Geometry check sheet. Reference: the model listing, model coordinates, mm. Face numbers are marked on the shaded views. A direction names the side the tool comes from. Give positions to 0.01 mm unless a question says otherwise; leave off trailing zeros. Order: outer loops, then holes, each group sorted by start corner. A loop starts at its lowest first (then second) coordinate and runs counter-clockwise, first axis right, second up. Notation, with made-up numbers: M 76.25,-9 L 87.25,-9 A17 ccw 87.25,9 Z; hole C 5,52.5 d10. An arc over 180 degrees is marked long. Put each result on its own line as item: value. Start each with the question number.
Q1. Material ranges on L1, parallel to Y at x = 0, z = 4.75; L2, parallel to Y at x = -2, z = 4.5; L3, parallel to X at y = 1, z = 4.25, recorded low to high.
Q2. Mould release check, pull along X, two halves, no side actions. Record for the marked faces 3, 4 and 5: +X half, -X half, draft (parallel to the pull), parting line (faces both ways), or undercut.
Q3. Section check B-B on y = 0. Record the cut outline in (x, z).
Q4. Access from +Z, -Z, +X, -X, +Y, -Y to the whole of each face (thin tool, end or side, straight path). Record for the marked faces 1 and 2.
Q5. Go/stop test with flat-tipped pins: pin 1 (5 mm diameter, centred on x = -5, z = 2.5, fed in from -Y); pin 2 (1.5 mm diameter, centred on y = 1, z = 3, fed in from -X); pin 3 (4 mm diameter, centred on x = 4, y = 4.5, fed in from +Z). Record where each tip stops, or that it passes through.
Q6. Section check D-D on z = 20. Record the cut outline in (x, y).
Q7. Section check A-A on z = 7.75. Record the cut outline in (x, y).
```python
from build123d import *

# Parameters (mm, degrees)
F0_R     = 5.25
F1_DEPTH = 11.7
F2_R     = 8.9
F3_DEPTH = 1.5
F4_R     = 3.4
F5_DEPTH = 9.5
F7_R     = 0.0965685425
F8_R     = 3.4
F9_DEPTH = 11.8
F10_R    = 1.4485281374


# Not quite as in the source:
# - a fillet or chamfer that OpenCascade refuses, or shapes differently, is made with other operations: its cross-section is extruded or revolved along the edge and cut away or added


with BuildPart() as f1:
    # F0 (on Top) → F1 (new body)
    with BuildSketch(Plane.XY):
        Circle(F0_R)
    extrude(amount=F1_DEPTH)

    # F2 (on face) → F3 (join)
    with BuildSketch(Plane.XY.offset(11.7)):
        Circle(F2_R)
    extrude(amount=F3_DEPTH)

    # F4 (on face) → F5 (join)
    with BuildSketch(Plane.XY.offset(13.2)):
        Circle(F4_R)
    extrude(amount=F5_DEPTH)

    # F6: fillet of radius 5 on 1 edges, made by hand

    # F6_s1 → F6_t2 (revolve, cut)
    with BuildSketch(Plane.XZ):
        with BuildLine():
            ThreePointArc((8.9, 11.7), (7.2657774588, 12.8097722286), (5.3292857857, 13.2))
            Line((5.3292857857, 13.2), (8.9, 13.2))
            Line((8.9, 13.2), (8.9, 11.7))
        make_face()
    revolve(axis=Axis((0, 0, 13.2), (0, 0, 1)), mode=Mode.SUBTRACT)

    # F7
    f7_edges = [f1.edges().sort_by_distance(p)[0] for p in [
        (3.4, 0, 17.95),
        (-3.4, 0, 13.2),
        (-3.4, 0, 22.7),
    ]]
    fillet(f7_edges, radius=F7_R)

    # F8 (on face) → F9 (cut)
    with BuildSketch(Plane(origin=(0, 0, 0), x_dir=(1, 0, 0), z_dir=(0, 0, -1))):
        Circle(F8_R)
    extrude(amount=-F9_DEPTH, mode=Mode.SUBTRACT)

    # F10
    f10_edges = [f1.edges().sort_by_distance(p)[0] for p in [
        (-5.25, 0, 0),
    ]]
    fillet(f10_edges, radius=F10_R)


solid = f1.part
```
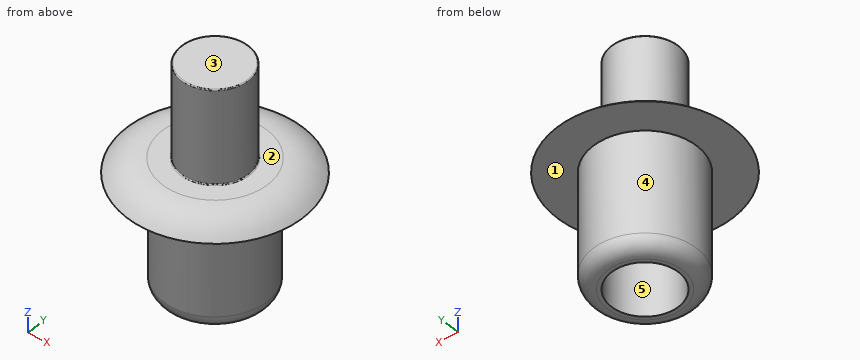
Results found:
1. L1: y = -5.25 to -3.4, 3.4 to 5.25
1. L2: y = -4.85 to -2.75, 2.75 to 4.85
1. L3: x = -5.15 to -3.25, 3.25 to 5.15
2. face 3: draft
2. face 4: parting line
2. face 5: undercut
3. outline: M -8.9,11.7 L -5.25,11.7 L -5.25,1.45 A1.45 ccw -3.8,0 L -3.4,0 L -3.4,11.8 L 3.4,11.8 L 3.4,0 L 3.8,0 A1.45 ccw 5.25,1.45 L 5.25,11.7 L 8.9,11.7 A5 ccw 5.33,13.2 L 3.5,13.2 A0.1 cw 3.4,13.3 L 3.4,22.6 A0.1 ccw 3.3,22.7 L -3.3,22.7 A0.1 ccw -3.4,22.6 L -3.4,13.3 A0.1 cw -3.5,13.2 L -5.33,13.2 A5 ccw Z
4. face 1: -Z
4. face 2: +Z
5. pin 1: stops at y = -4.62
5. pin 2: stops at x = -5.24
5. pin 3: stops at z = 13.2
6. outline: C 0,0 d6.8
7. outline: C 0,0 d10.5; hole C 0,0 d6.8
